The drawing under review shows one solid part. Ordinate dimensions are in mm from its lowest x, y, z. A direction names the side the tool comes from. Coordinates: 2 decimals unless noted, no trailing zeros. Loops run counter-clockwise (first coordinate to the right, second up) from the corner with the lowest first, then second, coordinate; pieces in that order, holes last. Notation, with made-up numbers: M 12,83.25 L 44,83.25 A28 cw 44,104.25 Z; hole C 34,68.5 d8. An arc over 180 degrees is marked long. Return JSON: item names as keys, results as strings.
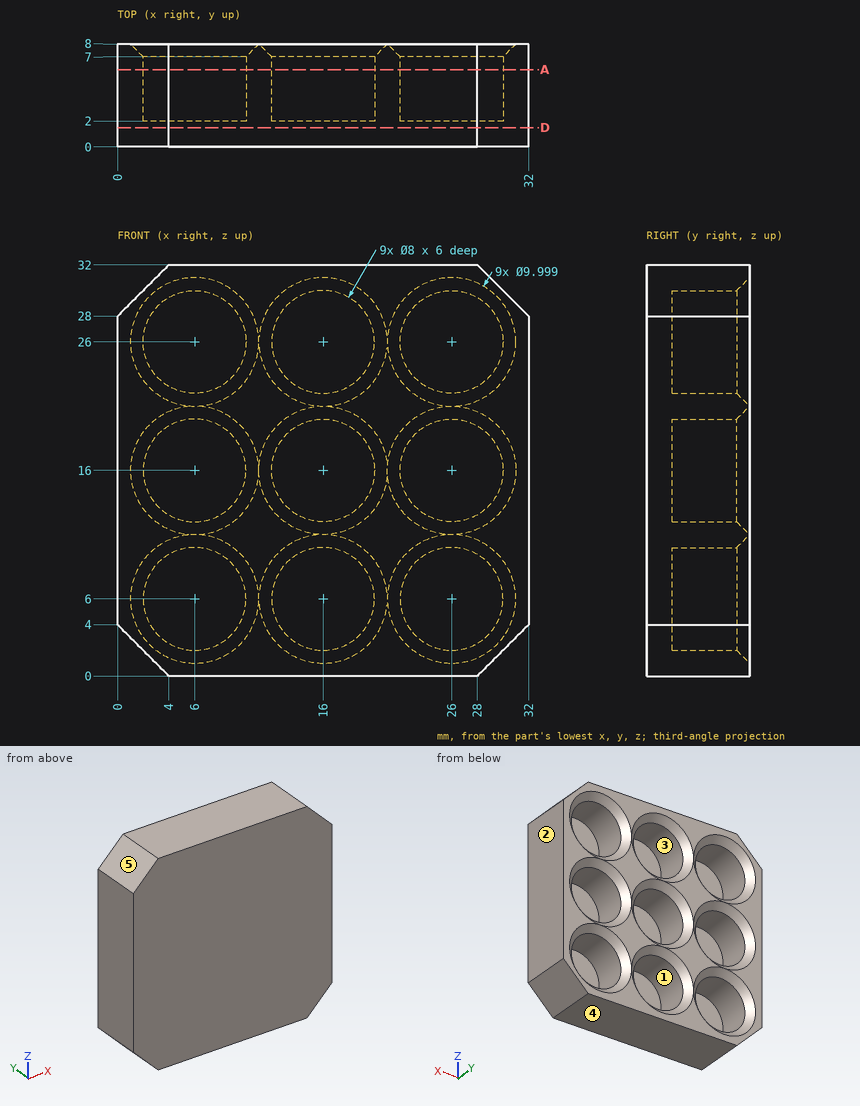
1. To check wall thickness, follow line 1 (Z direction, x = 26, y = 4.8); line 2 (Z direction, x = 4.5, y = 7.5) (1 decimal). State the ranges of each line that lie inside material, in increasing order.
Check values:
{"line 1": "0 to 2, 10 to 12, 20 to 22, 30 to 32", "line 2": "0 to 1.8, 10.2 to 11.8, 20.2 to 21.8, 30.2 to 32"}
2. Add section D-D on y = 1.5. Give the boundary of the cut face in (x, z), plus the area to 3 significant figures.
Check values:
{"outline": "M 0,4 L 4,0 L 28,0 L 32,4 L 32,28 L 28,32 L 4,32 L 0,28 Z", "area": "992 mm²"}
3. The part is to be moulded in two halves that separate along X. For the marked faces 3, 4 and 5, say which applies: released by +X, released by -X, zero draft, split by the parting line, or undercut.
Check values:
{"face 3": "undercut", "face 4": "zero draft", "face 5": "released by -X"}
4. Add section A-A on y = 6. State how many separate pieces and enclosed holes the cut face has.
Check values:
{"separate pieces": "1", "enclosed holes": "9"}
5. Machinability: for the marked faces 1 and 2, which of the approach directions +Z, -Z, +X, -X, +Y, -Y give a long, thin tool a straight path to every point of the face, cutting with its end or side? Answer none if there is none.
Check values:
{"face 1": "+Y", "face 2": "+Z, -Z, +X, +Y, -Y"}
6. Insertion check: pin 1 Ø10.5 at (x, z) = (26, 26) entering from -Y; pin 2 Ø6.5 at (x, z) = (5.5, 6) entering from +Y; pin 3 Ø9 at (x, z) = (6, 26) entering from +Y; pin 4 Ø6.5 at (x, z) = (26, 4.5) entering from +Y. Each pin has a flat end and moves straight along its axis. Give the tip position at first contact, or say it passes through.
Check values:
{"pin 1": "y = 0", "pin 2": "y = 2", "pin 3": "y = 7.5", "pin 4": "y = 7.75"}
